Part print with two shaded views. Sizes in mm from the minimum x, y, z corner. A direction names the side the tool comes from. Round coordinates to 2 decimals unless told otherwise and drop trailing zeros. Write each loop counter-clockwise with the first axis right and the second up, starting at its lowest first coordinate (ties: lowest second). Pieces come first, ordered by that corner, then holes.
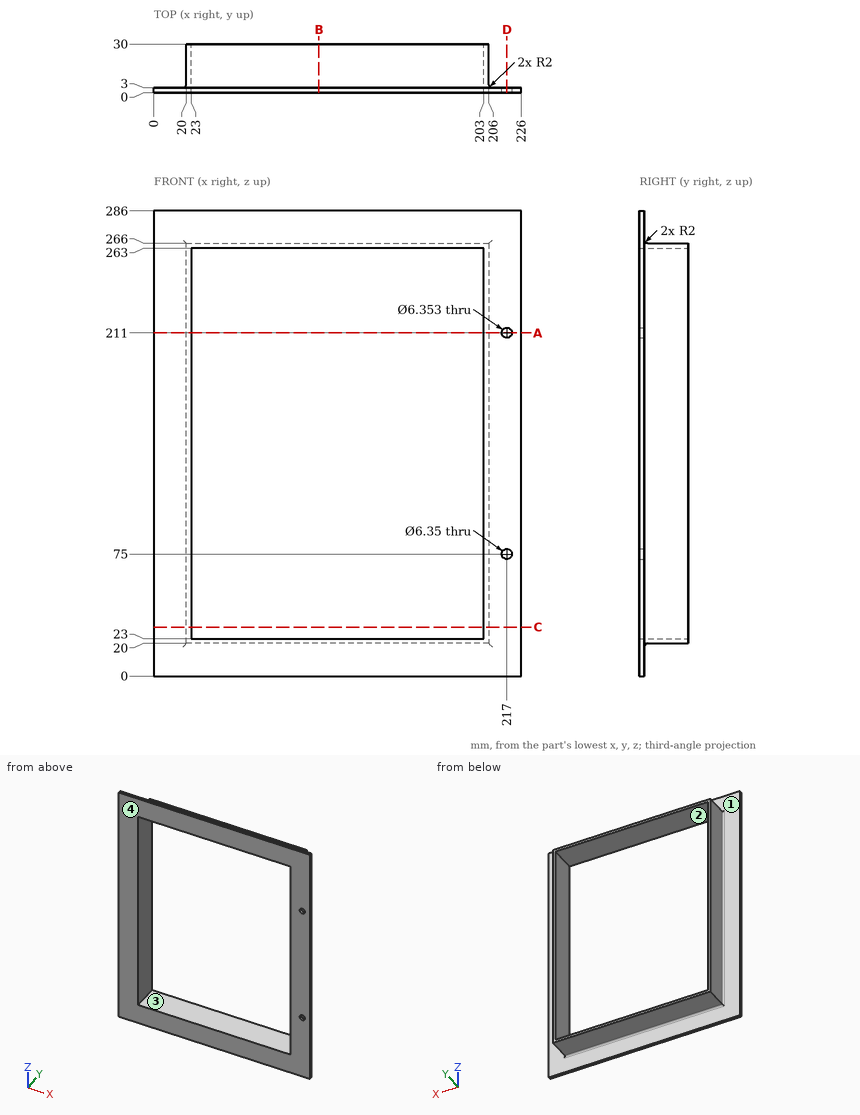
Q1. Drop flat-ended pins along their axis: pin 1 (2 mm diameter, centred on x = 198.5, y = 14.5, fed in from +Z); pin 2 (5 mm diameter, centred on y = 16, z = 231, fed in from +X); pin 3 (12.5 mm diameter, centred on x = 156, y = 21, fed in from -Z). Give the stop position or say it passes through.
Values follow:
pin 1: stops at z = 266
pin 2: stops at x = 206
pin 3: stops at z = 20
Q2. Which spindle directions (+Z, -Z, +X, -X, +Y, -Y) get a long thin tool onto all of the face, cutting with end or side? Do the marked faces 3 and 4. Say none if no direction does.
Values follow:
face 3: +Y, -Y
face 4: +Z, -Z, +X, -X, -Y
Q3. Cut at C-C on z = 30. Write the cut outline in (x, y).
Values follow:
outline: (0, 0) - (23, 0) - (23, 30) - (20, 30) - (20, 5) arc R2 cw to (18, 3) - (0, 3) - close; (203, 0) - (226, 0) - (226, 3) - (208, 3) arc R2 cw to (206, 5) - (206, 30) - (203, 30) - close
Q4. Cut at B-B on x = 101.5. Write the cut outline in (y, z), plus the area to 3 significant figures.
Values follow:
outline: (0, 0) - (3, 0) - (3, 18) arc R2 cw to (5, 20) - (30, 20) - (30, 23) - (0, 23) - close; (0, 263) - (30, 263) - (30, 266) - (5, 266) arc R2 cw to (3, 268) - (3, 286) - (0, 286) - close
area: 302 mm2
Q5. Wall check: L1, parallel to X at y = 1.5, z = 211; L2, parallel to Z at x = 217, y = 1.3 (1 decimal); L3, parallel to Z at x = 168, y = 10.5. Give the ranges that are in metal, low to high.
Values follow:
L1: x = 0 to 23, 203 to 213.82, 220.18 to 226
L2: z = 0 to 71.8, 78.2 to 207.8, 214.2 to 286
L3: z = 20 to 23, 263 to 266
Q6. Cut at D-D on x = 217. Write the cut outline in (y, z) (1 decimal).
Values follow:
outline: (0, 0) - (3, 0) - (3, 71.8) - (0, 71.8) - close; (0, 78.2) - (3, 78.2) - (3, 207.8) - (0, 207.8) - close; (0, 214.2) - (3, 214.2) - (3, 286) - (0, 286) - close
Q7. Cut at A-A on z = 211. Write the cut outline in (x, y).
Values follow:
outline: (0, 0) - (23, 0) - (23, 30) - (20, 30) - (20, 5) arc R2 cw to (18, 3) - (0, 3) - close; (203, 0) - (213.82, 0) - (213.82, 3) - (208, 3) arc R2 cw to (206, 5) - (206, 30) - (203, 30) - close; (220.18, 0) - (226, 0) - (226, 3) - (220.18, 3) - close
Q8. Mould opens along Z. For the marked faces 1 and 2 say: +Z half, -Z half, draft (parallel to the pull), parting line (faces both ways), or undercut.
Values follow:
face 1: draft
face 2: undercut
